Geometry: final body of the model. Coordinates: model frame, mm. Give positions to 0.01 mm unless a question says otherwise; leave off trailing zeros. Loops run counter-clockwise (first coordinate to the right, second up) from the corner with the lowest first, then second, coordinate; pieces in that order, holes last. Notation, with made-up numbers: (21, -12) -> (72, -12) arc R7 ccw to (72, -8) -> close; hole circle Ø8 at (55.5, -10). An arc over 180 degrees is marked (long way). Answer in a Markdown table with one row per item. Add a question column.
1) Section query A-A (x = 0). Return the cut outline in (y, z), plus the area to 3 significant figures.
2) First-contact query: P1, Ø4, axis at x = -12.5, y = 0, coming from the +Z side; P2, Ø3, axis at x = 14, y = -43.5, coming from the +Z side. Flat tips, straight axial feed; report the tip coordinate or a pass-through.
3) Line query: line 1 (Y direction, x = 0, z = 0.5); line 2 (X direction, y = 10.5, z = 2.6); line 3 (X direction, y = 35, z = 1.75). Output: solid intervals per line, ascending. Write a range as from..to.
4) Section query D-D (x = -7). Return the cut outline in (y, z), plus the area to 3 significant figures.
5) Draft query along X for faces 1 (the cylindrical face through (14.8, 37, 1.5)), 2 (the flat face through (-29.75, 1, 1)), 3 (the flat face through (0, 46, 1)), 4 (the flat face through (29.75, 1, 1)). Return one class per face: +X half, -X half, draft (parallel to the pull), parting line (faces both ways), or undercut.
6) Section query C-C (z = 0.65). Give the number of separate pieces and of enclosed holes in the cut face, plus the area to 3 significant figures.
7) Section query B-B (y = 35.5). Return the cut outline in (x, z), plus the area to 3 significant figures.
Autodesk Fusion 360 part; units mm, degrees
sketch "Sketch1" plane through (0, 0, 0) normal (0, 0, 1) x (1, 0, 0)
  circle A0 centre (0, 0) radius 29.75
  circle A1 centre (0, 0) radius 12.5
  circle A2 centre (0, 0) radius 15
  circle A3 centre (0, 12.5) radius 1.7
  circle A4 centre (-10.6066, 10.6066) radius 1.7
  circle A5 centre (-10.6066, -10.6066) radius 1.7
  circle A6 centre (-12.5, 0) radius 1.7
  circle A7 centre (10.6066, -10.6066) radius 1.7
  circle A8 centre (0, -12.5) radius 1.7
  circle A9 centre (10.6066, 10.6066) radius 1.7
  circle A10 centre (12.5, 0) radius 1.7
  circle A11 centre (-14, 35.5) radius 1.7
  circle A12 centre (14, 35.5) radius 1.7
  circle A13 centre (14, -35.5) radius 1.7
  circle A14 centre (-14, -35.5) radius 1.7
  line L0 (29.75, 38) -> (29.75, -38)
  line L1 (-29.75, -38) -> (-29.75, 38)
  circle A15 centre (0, 0) radius 9
  line L2 (29.75, 38) -> (29.75, 46)
  line L3 (29.75, 46) -> (-29.75, 46)
  line L4 (-29.75, 46) -> (-29.75, 38)
  circle A16 centre (-14, 43.5) radius 1.7
  circle A17 centre (14, 43.5) radius 1.7
  line L5 (-29.75, -46) -> (29.75, -46)
  line L6 (29.75, -46) -> (29.75, -38)
  line L7 (-29.75, -38) -> (-29.75, -46)
  circle A18 centre (-14, -43.5) radius 1.7
  circle A19 centre (14, -43.5) radius 1.7
  dimension "d1" = 59.5
  dimension "d2" = 25
  dimension "d3" = 30
  dimension "d5" = 3.4
  dimension "d10" = 360
  dimension "d13" = 3.4
  dimension "d14" = 3.4
  dimension "d15" = 3.4
  dimension "d16" = 3.4
  dimension "d17" = 59.5
  dimension "d18" = 76
  dimension "d19" = 18
  dimension "d23" = 8
  dimension "d24" = 3.4
  dimension "d25" = 3.4
  dimension "d27" = 59.5
  dimension "d28" = 8
  dimension "d29" = 3.4
  dimension "d30" = 3.4
extrude "Extrude2" add sketch "Sketch1" along normal blind 3 contours A0 | A0 L0 L1 L5 L6 L7 | A0 L0 L1 L2 L3 L4 | A1 A3 A6 A8 A10 | A2 A4 A5 A7 A9
Evaluation:
| question | item | result |
|---|---|---|
| 1 | outline | (-46, 0) -> (-14.2, 0) -> (-14.2, 3) -> (-46, 3) -> close; (-10.8, 0) -> (-9, 0) -> (-9, 3) -> (-10.8, 3) -> close; (9, 0) -> (10.8, 0) -> (10.8, 3) -> (9, 3) -> close; (14.2, 0) -> (46, 0) -> (46, 3) -> (14.2, 3) -> close |
| 1 | area | 202 mm² |
| 2 | P1 | z = 3 |
| 2 | P2 | through |
| 3 | line 1 | -46..-14.2, -10.8..-9, 9..10.8, 14.2..46 |
| 3 | line 2 | -29.75..-12.3, -8.91..8.91, 12.3..29.75 |
| 3 | line 3 | -29.75..-15.62, -12.38..12.38, 15.62..29.75 |
| 4 | outline | (-46, 0) -> (-5.66, 0) -> (-5.66, 3) -> (-46, 3) -> close; (5.66, 0) -> (46, 0) -> (46, 3) -> (5.66, 3) -> close |
| 4 | area | 242 mm² |
| 5 | face 1 | undercut |
| 5 | face 2 | -X half |
| 5 | face 3 | draft |
| 5 | face 4 | +X half |
| 6 | separate pieces | 1 |
| 6 | enclosed holes | 17 |
| 6 | area | 5,070 mm² |
| 7 | outline | (-29.75, 0) -> (-15.7, 0) -> (-15.7, 3) -> (-29.75, 3) -> close; (-12.3, 0) -> (12.3, 0) -> (12.3, 3) -> (-12.3, 3) -> close; (15.7, 0) -> (29.75, 0) -> (29.75, 3) -> (15.7, 3) -> close |
| 7 | area | 158 mm² |
